The model under review builds one solid part; all positions refer to its coordinate system, in mm. Round coordinates to 2 decimals unless told otherwise and drop trailing zeros. Write each loop counter-clockwise with the first axis right and the second up, starting at its lowest first coordinate (ties: lowest second). Pieces come first, ordered by that corner, then holes. Notation, with made-up numbers: (-34, 1) - (-10, 1) arc R26 cw to (-10, 25) - close; hole circle Ø5 at (82.5, 11.25). An arc over 180 degrees is marked (long way). Use one line per item in the form item = value.
from build123d import *

# Parameters (mm, degrees)
SKETCH1_R           = 16.5
BOSS_EXTRUDE1_DEPTH = 4
SKETCH2_R           = 0.75
CUT_EXTRUDE1_DEPTH  = 24.674881204


with BuildPart() as part:
    # Sketch1 → Boss-Extrude1 (new body)
    with BuildSketch(Plane.XY):
        Circle(SKETCH1_R)
    extrude(amount=BOSS_EXTRUDE1_DEPTH)

    # Sketch2 → Cut-Extrude1 (cut, through all)
    with BuildSketch(Plane.XY.offset(4)):
        with Locations((0, 9.166448404)):
            Circle(SKETCH2_R)
        with Locations((7.93837718, 4.583224202)):
            Circle(SKETCH2_R)
        with Locations((7.93837718, -4.583224202)):
            Circle(SKETCH2_R)
        with Locations((0, -9.166448404)):
            Circle(SKETCH2_R)
        with Locations((-7.93837718, -4.583224202)):
            Circle(SKETCH2_R)
        with Locations((-7.93837718, 4.583224202)):
            Circle(SKETCH2_R)
        with Locations((0, 4.583224202)):
            Circle(SKETCH2_R)
        with Locations((4.358905243, 1.416294167)):
            Circle(SKETCH2_R)
        with Locations((2.693951594, -3.707906268)):
            Circle(SKETCH2_R)
        with Locations((-2.693951594, -3.707906268)):
            Circle(SKETCH2_R)
        with Locations((-4.358905243, 1.416294167)):
            Circle(SKETCH2_R)
    extrude(amount=-CUT_EXTRUDE1_DEPTH, mode=Mode.SUBTRACT)


solid = part.part
(1) Insertion check: P1, Ø2, axis at x = 0, y = 9.17, coming from the -Z side; P2, Ø1.5, axis at y = -12, z = 2.5, coming from the -X side; P3, Ø1, axis at y = -8, z = 2.5, coming from the -X side. Each pin has a flat end and moves straight along its axis. Give the tip position at first contact, or say it passes through.
Geometry results:
P1 = 0
P2 = -12.07
P3 = -14.7
(2) The part is to be moulded in two halves that separate along Y. For faces 1 (the cylindrical face through (15.24, -6.32, 1.97)), 2 (the cylindrical face through (3.61, 1.45, 2.03)), 3 (the flat face through (0, 0, 4)), say which applies: +Y half, -Y half, draft (parallel to the pull), parting line (faces both ways), or undercut.
Geometry results:
face_1 = parting line
face_2 = undercut
face_3 = draft
(3) To check wall thickness, follow L1, parallel to Y at x = 0, z = 2.15; L2, parallel to X at y = 5, z = 2.2; L3, parallel to X at y = 4, z = 0.95. State the ranges of each line that lie inside material, in increasing order.
Geometry results:
L1 = -16.5 to -9.92, -8.42 to 3.83, 5.33 to 8.42, 9.92 to 16.5
L2 = -15.72 to -8.56, -7.31 to -0.62, 0.62 to 7.31, 8.56 to 15.72
L3 = -16.01 to -8.41, -7.47 to -0.47, 0.47 to 7.47, 8.41 to 16.01
(4) Add section B-B on z = 2.25. Count the separate pieces of the cut face and the enclosed holes in it, then the cut area to 3 significant figures.
Geometry results:
separate_pieces = 1
enclosed_holes = 11
area = 836 mm2
(5) Add section A-A on x = 0. Write out the cut boundary in (y, z), then the cut area to 3 significant figures.
Geometry results:
outline = (-16.5, 0) - (-9.92, 0) - (-9.92, 4) - (-16.5, 4) - close; (-8.42, 0) - (3.83, 0) - (3.83, 4) - (-8.42, 4) - close; (5.33, 0) - (8.42, 0) - (8.42, 4) - (5.33, 4) - close; (9.92, 0) - (16.5, 0) - (16.5, 4) - (9.92, 4) - close
area = 114 mm2
(6) Add section D-D on x = -9.5. Write out the cut boundary in (y, z), then the cut area to 3 significant figures.
Geometry results:
outline = (-13.49, 0) - (13.49, 0) - (13.49, 4) - (-13.49, 4) - close
area = 108 mm2
(7) Add section C-C on y = 10.5. Write out the cut boundary in (x, z).
Geometry results:
outline = (-12.73, 0) - (12.73, 0) - (12.73, 4) - (-12.73, 4) - close
